from build123d import *

# Parameters (mm, degrees)
SKETCH_1_R          = 1.25
EXTRUDE_1_DEPTH     = 3
SKETCH_2_R          = 2.5
CUT_EXTRUDE_1_DEPTH = 12


with BuildPart() as part:
    # 草图1 → 凸台-拉伸1 (new body)
    with BuildSketch(Plane.XY):
        with BuildLine():
            Line((-14, 25), (-22.127465978, 25))
            ThreePointArc((-22.127465978, 25), (-23.607464398, 23.607464398), (-25, 22.127465978))
            Line((-25, 22.127465978), (-25, 14))
            ThreePointArc((-25, 14), (-15.100505063, 9.899494937), (-11, 0))
            ThreePointArc((-11, 0), (-15.100505063, -9.899494937), (-25, -14))
            Line((-25, -14), (-25, -22.127465978))
            ThreePointArc((-25, -22.127465978), (-23.607464398, -23.607464398), (-22.127465978, -25))
            Line((-22.127465978, -25), (-14, -25))
            ThreePointArc((-14, -25), (0, -11), (14, -25))
            Line((14, -25), (22.127465978, -25))
            ThreePointArc((22.127465978, -25), (23.607464398, -23.607464398), (25, -22.127465978))
            Line((25, -22.127465978), (25, -14))
            ThreePointArc((25, -14), (11, 0), (25, 14))
            Line((25, 14), (25, 22.127465978))
            ThreePointArc((25, 22.127465978), (23.607464398, 23.607464398), (22.127465978, 25))
            Line((22.127465978, 25), (14, 25))
            ThreePointArc((14, 25), (0, 11), (-14, 25))
        make_face()
        with Locations((-21.25, -21.25)):
            Circle(SKETCH_1_R, mode=Mode.SUBTRACT)
        with Locations((21.25, -21.25)):
            Circle(SKETCH_1_R, mode=Mode.SUBTRACT)
        with Locations((-21.25, 21.25)):
            Circle(SKETCH_1_R, mode=Mode.SUBTRACT)
        with Locations((21.25, 21.25)):
            Circle(SKETCH_1_R, mode=Mode.SUBTRACT)
    extrude(amount=EXTRUDE_1_DEPTH)

    # 草图2 → 切除-拉伸1 (cut)
    with BuildSketch(Plane.XY.offset(3)):
        with BuildLine():
            ThreePointArc((20.291287847, 25), (18, 26.5), (15.708712153, 25))
            Line((15.708712153, 25), (20.291287847, 25))
        make_face()
        with BuildLine():
            Line((20.291287847, 25), (15.708712153, 25))
            ThreePointArc((15.708712153, 25), (17.489225891, 21.552734218), (20.5, 24))
            ThreePointArc((20.5, 24), (20.447265782, 24.510774109), (20.291287847, 25))
        make_face()
        with BuildLine():
            ThreePointArc((20.5, -24), (17.489225891, -21.552734218), (15.708712153, -25))
            Line((15.708712153, -25), (20.291287847, -25))
            ThreePointArc((20.291287847, -25), (20.447265782, -24.510774109), (20.5, -24))
        make_face()
        with BuildLine():
            Line((20.291287847, -25), (15.708712153, -25))
            ThreePointArc((15.708712153, -25), (18, -26.5), (20.291287847, -25))
        make_face()
        with Locations((-18, 24)):
            Circle(SKETCH_2_R)
        with Locations((-18, -24)):
            Circle(SKETCH_2_R)
    extrude(amount=-CUT_EXTRUDE_1_DEPTH, mode=Mode.SUBTRACT)


solid = part.part
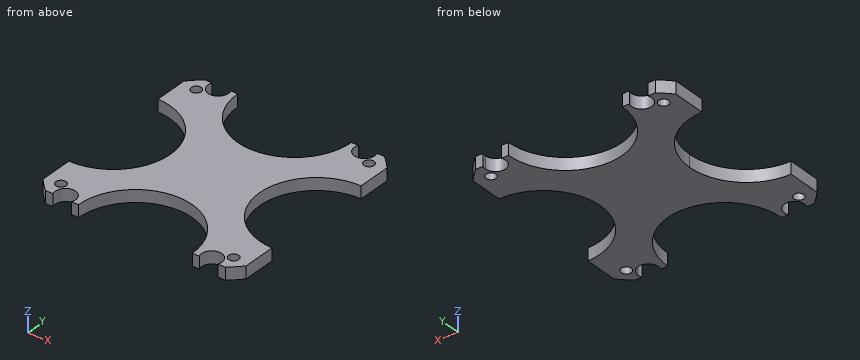
Read the model definition and answer for the solid it produces. Units are mm, in the model's axes. Round coordinates to 2 decimals unless told otherwise and drop trailing zeros. Write each loop counter-clockwise with the first axis right and the second up, starting at its lowest first coordinate (ties: lowest second). Pieces come first, ordered by that corner, then holes.
Q1. Straight lines are drawn through the part: line 1 (Y direction, x = -21.25, z = 2.2); line 2 (X direction, y = 24, z = 2); line 3 (Y direction, x = -19, z = 2). For each, find the intervals that lie inside material, in ascending order.
Values:
line 1: y = -25 to -22.5, -20 to -13.49, 13.49 to 20, 22.5 to 25
line 2: x = -23.21 to -20.5, -15.5 to -13.96, 13.96 to 15.5, 20.5 to 23.21
line 3: y = -21.71 to -12.65, 12.65 to 21.71
Q2. Flat-ended cylindrical pins translate along their axes: P1, Ø2, axis at x = -21.25, y = -21.25, coming from the +Z side; P2, Ø4, axis at x = 21.25, y = 21.25, coming from the +Z side; P3, Ø1.5, axis at y = -4.5, z = 1.5, coming from the -X side; P4, Ø1.5, axis at x = 6, z = 1.5, coming from the -Y side. Find the tip coordinate at first contact, or state that the pin passes through.
Values:
P1: passes through
P2: stops at z = 3
P3: stops at x = -12.02
P4: stops at y = -12.73
Q3. Find section B-B on y = 15. Determine the outline of the cut face in (x, z), and give its area (3 significant figures).
Values:
outline: (-25, 0) - (-9.8, 0) - (-9.8, 3) - (-25, 3) - close; (9.8, 0) - (25, 0) - (25, 3) - (9.8, 3) - close
area: 91.2 mm2
Q4. Find section C-C on z = 2.1. Determine the outline of the cut face in (x, y), and give its area (3 significant figures).
Values:
outline: (-25, -22.13) arc R33.39 ccw to (-22.13, -25) - (-20.29, -25) arc R2.5 cw (long way) to (-15.71, -25) - (-14, -25) arc R14 cw to (14, -25) - (15.71, -25) arc R2.5 cw (long way) to (20.29, -25) - (22.13, -25) arc R33.39 ccw to (25, -22.13) - (25, -14) arc R14 cw to (25, 14) - (25, 22.13) arc R33.39 ccw to (22.13, 25) - (20.29, 25) arc R2.5 cw (long way) to (15.71, 25) - (14, 25) arc R14 cw to (-14, 25) - (-15.71, 25) arc R2.5 cw (long way) to (-20.29, 25) - (-22.13, 25) arc R33.39 ccw to (-25, 22.13) - (-25, 14) arc R14 cw to (-25, -14) - close; hole circle Ø2.5 at (-21.25, -21.25); hole circle Ø2.5 at (-21.25, 21.25); hole circle Ø2.5 at (21.25, -21.25); hole circle Ø2.5 at (21.25, 21.25)
area: 1,170 mm2
Q5. Find section A-A on x = -18. Determine the outline of the cut face in (y, z).
Values:
outline: (-21.5, 0) - (-12.12, 0) - (-12.12, 3) - (-21.5, 3) - close; (12.12, 0) - (21.5, 0) - (21.5, 3) - (12.12, 3) - close
Q6. Find section D-D on x = 21.25. Determine the outline of the cut face in (y, z).
Values:
outline: (-25, 0) - (-22.5, 0) - (-22.5, 3) - (-25, 3) - close; (-20, 0) - (-13.49, 0) - (-13.49, 3) - (-20, 3) - close; (13.49, 0) - (20, 0) - (20, 3) - (13.49, 3) - close; (22.5, 0) - (25, 0) - (25, 3) - (22.5, 3) - close
